from build123d import *

# Parameters (mm, degrees)
SKETCH1_W           = 55.95
SKETCH1_H           = 4.95
BOSS_EXTRUDE1_DEPTH = 2.5
SKETCH2_W           = 30
SKETCH2_H           = 30
BOSS_EXTRUDE2_DEPTH = 2.5
SKETCH3_W           = 30
SKETCH3_H           = 30
SKETCH3_W_2         = 23.15
SKETCH3_H_2         = 22.65
BOSS_EXTRUDE3_DEPTH = 2.5
SKETCH4_W           = 3
SKETCH4_H           = 9
CUT_EXTRUDE1_DEPTH  = 236.857029442
FILLET1_R           = 2
SKETCH5_W           = 4.971025799
SKETCH5_H           = 15.475
SKETCH5_W_2         = 5
BOSS_EXTRUDE4_DEPTH = 5
FILLET2_R           = 2
SKETCH6_W           = 3
SKETCH6_H           = 11
CUT_EXTRUDE2_DEPTH  = 236.857029442


with BuildPart() as part:
    # Sketch1 → Boss-Extrude1 (new body)
    with BuildSketch(Plane(origin=(0, 0, 0), x_dir=(1, 0, 0), z_dir=(0, 1, 0))):
        with Locations((79.200782246, 194.508385484)):
            Rectangle(SKETCH1_W, SKETCH1_H)
    extrude(amount=BOSS_EXTRUDE1_DEPTH)

    # Sketch2 → Boss-Extrude2 (add)
    with BuildSketch(Plane(origin=(0, 0, 0), x_dir=(1, 0, 0), z_dir=(0, 1, 0))):
        with Locations((78.650782246, 195.084840094)):
            Rectangle(SKETCH2_W, SKETCH2_H)
    extrude(amount=BOSS_EXTRUDE2_DEPTH)

    # Sketch3 → Boss-Extrude3 (add)
    with BuildSketch(Plane.XZ):
        with Locations((78.650782246, -195.084840094)):
            Rectangle(SKETCH3_W, SKETCH3_H)
        with Locations((79.200782246, -194.508385484)):
            Rectangle(SKETCH3_W_2, SKETCH3_H_2, mode=Mode.SUBTRACT)
    extrude(amount=BOSS_EXTRUDE3_DEPTH)

    # Sketch4 → Cut-Extrude1 (cut, through all)
    with BuildSketch(Plane.XZ):
        with Locations((72.475782246, -194.693385484)):
            Rectangle(SKETCH4_W, SKETCH4_H)
    extrude(amount=-CUT_EXTRUDE1_DEPTH, mode=Mode.SUBTRACT)

    # Fillet1
    fillet1_edges = [part.edges().sort_by_distance(p)[0] for p in [
        (63.650782246, 0, -210.084840094),
        (93.650782246, 0, -180.084840094),
        (63.650782246, 0, -180.084840094),
        (93.650782246, 0, -210.084840094),
    ]]
    fillet(fillet1_edges, radius=FILLET1_R)

    # Sketch5 → Boss-Extrude4 (add)
    with BuildSketch(Plane(origin=(0, 2.5, 0), x_dir=(1, 0, 0), z_dir=(0, 1, 0))):
        with Locations((61.165269347, 194.796612789)):
            Rectangle(SKETCH5_W, SKETCH5_H)
        with Locations((96.150782246, 194.796612789)):
            Rectangle(SKETCH5_W_2, SKETCH5_H)
    extrude(amount=-BOSS_EXTRUDE4_DEPTH)

    # Fillet2
    fillet2_edges = [part.edges().sort_by_distance(p)[0] for p in [
        (98.650782246, 0, -194.508385484),
        (58.679756447, 0, -194.508385484),
        (58.679756447, 0, -187.059112789),
        (58.679756447, 1.25, -192.033385484),
        (58.679756447, 1.25, -196.983385484),
        (58.679756447, 0, -202.534112789),
        (98.650782246, 0, -202.534112789),
        (98.650782246, 1.25, -192.033385484),
        (98.650782246, 1.25, -196.983385484),
        (98.650782246, 0, -187.059112789),
    ]]
    fillet(fillet2_edges, radius=FILLET2_R)

    # Sketch6 → Cut-Extrude2 (cut, through all)
    with BuildSketch(Plane.XZ):
        with Locations((85.975782246, -194.223385484)):
            Rectangle(SKETCH6_W, SKETCH6_H)
    extrude(amount=-CUT_EXTRUDE2_DEPTH, mode=Mode.SUBTRACT)


solid = part.part
Part model, mm, in its own coordinate system. A direction names the side the tool comes from. Coordinates: 2 decimals unless noted, no trailing zeros. Write each loop counter-clockwise with the first axis right and the second up, starting at its lowest first coordinate (ties: lowest second). Pieces come first, ordered by that corner, then holes. Notation, with made-up numbers: (67.25, -4) - (79.25, -4) arc R19 ccw to (79.25, 12) - close; hole circle Ø5 at (66, -18.75). An arc over 180 degrees is marked (long way). Put each result on its own line as item: value.
1. Band-saw the part on A-A (z = -194.25). Write the cut outline in (x, y).
Final values:
outline: (51.23, 0) - (56.68, 0) arc R2 cw to (58.68, -2) - (58.68, -2.5) - (67.63, -2.5) - (67.63, 0) - (70.98, 0) - (70.98, 2.5) - (51.23, 2.5) - close; (73.98, 0) - (84.48, 0) - (84.48, 2.5) - (73.98, 2.5) - close; (87.48, 0) - (90.78, 0) - (90.78, -2.5) - (98.65, -2.5) - (98.65, -2) arc R2 cw to (100.65, 0) - (107.18, 0) - (107.18, 2.5) - (87.48, 2.5) - close
2. Band-saw the part on D-D (y = 1.7). Give the number of separate pieces and of enclosed holes in the cut face, then the cut area to 3 significant figures.
Final values:
separate pieces: 1
enclosed holes: 2
area: 1,070 mm²
3. 3-axis set-ups, long thin cutter, end or side, ignore diameter. For faces 1 (the flat face through (95, 0, -187.059)), 2 (the flat face through (58.68, -2.2, -196.5)), 3 (the flat face through (54, 0, -195)): which of +Z, -Z, +X, -X, +Y, -Y reach the whole face in a straight line?
Final values:
face 1: +Z, +X, +Y, -Y
face 2: -X, -Y
face 3: +Z, -Z, -X, -Y
4. Band-saw the part on C-C (z = -184.75). Write the cut outline in (x, y).
Final values:
outline: (63.65, -2.5) - (67.63, -2.5) - (67.63, 0) - (90.78, 0) - (90.78, -2.5) - (93.65, -2.5) - (93.65, 2.5) - (63.65, 2.5) - close
5. Flat gauge pins, fed straight in: pin 1 Ø3 at (x, y) = (104, 1.5) entering from +Z; pin 2 Ø1.5 at (y, z) = (0.5, -206.5) entering from -X; pin 3 Ø1.5 at (y, z) = (0, -204) entering from +X. Where does each tip first touch, or does it go through?
Final values:
pin 1: stops at z = -192.03
pin 2: stops at x = 63.65
pin 3: stops at x = 93.65
6. Two-plate mould, pull along Z, no slides. Class faces 4 (the flat face through (70.976, 1, -195)), 5 (the cylindrical face through (93.049, 0.035, -180.655)), 6 (the flat face through (63.651, 0, -205)): +Z half, -Z half, draft (parallel to the pull), parting line (faces both ways), or undercut.
Final values:
face 4: undercut
face 5: +Z half
face 6: draft
7. Probe line 1 along X through (y, z) = (0.9, -189.25); line 2 along X through (y, z) = (-2, -184.5); line 3 along Z through (x, y) = (90, -1). List the from-to ranges inside material, lowest first. Write a range as [from, to].
Final values:
line 1: x = [58.68, 84.48], [87.48, 98.65]
line 2: x = [63.65, 67.63], [90.78, 93.65]
line 3: z = [-210.08, -205.83], [-183.18, -180.08]
